Could you check a few things on this drawing? It's one solid part, dimensions in mm from its lowest x, y, z. Round coordinates to 2 decimals unless told otherwise and drop trailing zeros. Order: outer loops, then holes, each group sorted by start corner. A loop starts at its lowest first (then second) coordinate and runs counter-clockwise, first axis right, second up. Notation, with made-up numbers: M -4.75,82 L 5.25,82 A24 cw 5.25,97 Z; hole C 25.25,-30.5 d10. An arc over 180 degrees is marked long. Answer as CSV lines item,"result". Start each with the question number.
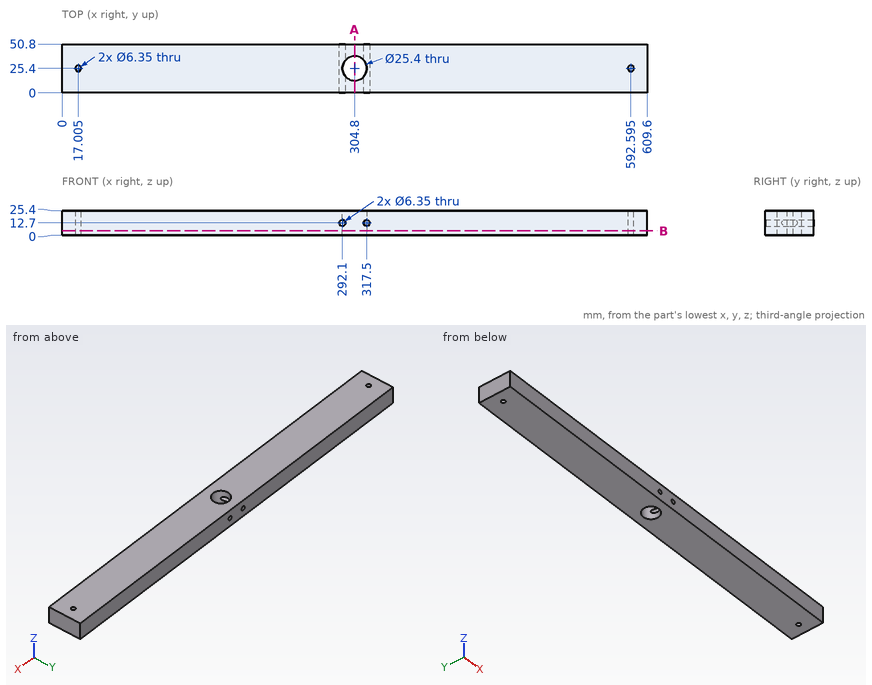
Item 1: If I drill on line 1 along X through (y, z) = (16.5, 14) (1 decimal); line 2 along X through (y, z) = (39.5, 15); line 3 along Z through (x, y) = (292.1, 33) (1 decimal), over which ranges is the centre line in solid material (lowest first)?
Item 2: If we section it at A-A on x = 304.8: Please give me the cut outline in (y, z).
Item 3: For P1, Ø10, axis at x = 292.1, z = 12.7, coming from the +Y side, with a flat end and sliding along its axis, tell me the tip position at first contact or that it passes through.
Item 4: If we section it at B-B on z = 4.5: Count the separate pieces of the cut face and the enclosed holes in it, and give its area (3 significant figures).
Geometry says:
1,line 1,"0 to 289.2, 295 to 295.7, 313.9 to 314.6, 320.4 to 609.6"
1,line 2,"0 to 289.91, 294.29 to 315.31, 319.69 to 609.6"
1,line 3,"0 to 9.5, 15.9 to 25.4"
2,outline,"M 0,0 L 12.7,0 L 12.7,25.4 L 0,25.4 Z; M 38.1,0 L 50.8,0 L 50.8,25.4 L 38.1,25.4 Z"
3,P1,"y = 50.8"
4,separate pieces,"1"
4,enclosed holes,"3"
4,area,"30,400 mm²"
